Work out the finished part from the listing and answer in its coordinate system (mm). Face numbers are marked on the shaded views. A direction names the side the tool comes from. Round coordinates to 2 decimals unless told otherwise and drop trailing zeros. Order: outer loops, then holes, each group sorted by start corner. A loop starts at its lowest first (then second) coordinate and runs counter-clockwise, first axis right, second up. Notation, with made-up numbers: M 58,38 L 70,38 A15 ccw 70,64 Z; hole C 51,15 d8. An arc over 180 degrees is marked long. Answer as a JSON object with one key per item and string values. Group by question number.
from build123d import *

# Parameters (mm, degrees)
BOSS_EXTRUDE1_DEPTH      = 4.15
BOSS_EXTRUDE1_DEPTH_BACK = 4.15
CUT_EXTRUDE1_DEPTH       = 6
CUT_EXTRUDE1_DEPTH_BACK  = 6
SKETCH2_W                = 10
SKETCH2_H                = 15
CUT_EXTRUDE2_DEPTH       = 2
BOSS_EXTRUDE2_DEPTH      = 2
BOSS_EXTRUDE2_DEPTH_BACK = 2
SKETCH5_W                = 4.4
SKETCH5_H                = 9
CUT_EXTRUDE3_DEPTH       = 3
CUT_EXTRUDE4_DEPTH       = 1
BOSS_EXTRUDE3_DEPTH      = 1
CUT_EXTRUDE5_DEPTH       = 3.2
SKETCH9_W                = 0.8
SKETCH9_H                = 0.8
CUT_EXTRUDE6_DEPTH       = 2.9
SKETCH10_W               = 0.8
SKETCH10_H               = 0.8
CUT_EXTRUDE7_DEPTH       = 2.9
SKETCH11_W               = 0.8
SKETCH11_H               = 0.8
CUT_EXTRUDE8_DEPTH       = 2.9
CUT_EXTRUDE9_DEPTH       = 2.9
CUT_EXTRUDE10_DEPTH      = 2.9
CUT_EXTRUDE11_DEPTH      = 2.9
CUT_EXTRUDE12_DEPTH      = 2.9
CUT_EXTRUDE13_DEPTH      = 2.9
CUT_EXTRUDE14_DEPTH      = 2.9
CUT_EXTRUDE15_DEPTH      = 1.1
BOSS_EXTRUDE4_DEPTH      = 3
BOSS_EXTRUDE4_DEPTH_BACK = 3
SKETCH20_R               = 0.65
BOSS_EXTRUDE5_DEPTH      = 10
SKETCH21_R               = 0.65
BOSS_EXTRUDE6_DEPTH      = 10
CUT_EXTRUDE16_DEPTH      = 3
CUT_EXTRUDE16_DEPTH_BACK = 3


with BuildPart() as part:
    # Sketch1 → Boss-Extrude1 (new, two sides: drawn at the far end of the back side and taken through both)
    with BuildSketch(Plane(origin=(0, 0, 0), x_dir=(0, 0, -1), z_dir=(1, 0, 0)).offset(-BOSS_EXTRUDE1_DEPTH_BACK)):
        with BuildLine():
            Line((-13, 1.4), (-13, -2.4))
            Line((-13, -2.4), (-12.8, -2.6))
            Line((-12.8, -2.6), (-9.85, -2.6))
            Line((-9.85, -2.6), (-9.1, -3.35))
            Line((-9.1, -3.35), (-4, -3.35))
            Line((-4, -3.35), (-4, -2.07))
            Line((-4, -2.07), (-2, -2.07))
            Line((-2, -2.07), (-2, -2.67))
            Line((-2, -2.67), (-0.5, -2.643817403))
            Line((-0.5, -2.643817403), (0, -2.509842806))
            Line((0, -2.509842806), (0, 2.069842806))
            Line((0, 2.069842806), (-0.5, 2.203817403))
            Line((-0.5, 2.203817403), (-2, 2.23))
            Line((-2, 2.23), (-2, 1.6))
            Line((-2, 1.6), (-4, 1.6))
            Line((-4, 1.6), (-4, 2.9))
            ThreePointArc((-4, 2.9), (-6.566392361, 2.777001893), (-9.1, 2.35))
            Line((-9.1, 2.35), (-9.85, 1.6))
            Line((-9.85, 1.6), (-12.8, 1.6))
            Line((-12.8, 1.6), (-13, 1.4))
        make_face()
    extrude(amount=BOSS_EXTRUDE1_DEPTH + BOSS_EXTRUDE1_DEPTH_BACK)

    # Sketch2 → Cut-Extrude1 (cut, two sides: drawn at the far end of the back side and taken through both)
    with BuildSketch(Plane(origin=(0, 0, 0), x_dir=(1, 0, 0), z_dir=(0, 1, 0)).offset(-CUT_EXTRUDE1_DEPTH_BACK)):
        with Locations((0, -6.5)):
            Rectangle(SKETCH2_W, SKETCH2_H)
        Polygon((-4.13, -9.1), (-3.38, -9.85), (-3.38, -12.8), (-3.18, -13), (3.18, -13), (3.38, -12.8), (3.38, -9.85), (4.13, -9.1), (4.13, -4), (3.185, -4), (3.185, -2), (3.8, -2), (3.773817403, -0.5), (3.639842806, 0), (-3.639842806, 0), (-3.773817403, -0.5), (-3.8, -2), (-3.185, -2), (-3.185, -4), (-4.13, -4), align=None, mode=Mode.SUBTRACT)
    extrude(amount=CUT_EXTRUDE1_DEPTH + CUT_EXTRUDE1_DEPTH_BACK, mode=Mode.SUBTRACT)

    # Sketch3 → Cut-Extrude2 (cut)
    with BuildSketch(Plane(origin=(0, 1.6, 0), x_dir=(1, 0, 0), z_dir=(0, 1, 0))):
        Polygon((-2.8, -4), (-2.8, -13), (2.8, -13), (2.8, -4), (2.04, -4), (2.04, 0), (-2.04, 0), (-2.04, -4), align=None)
    extrude(amount=CUT_EXTRUDE2_DEPTH, mode=Mode.SUBTRACT)

    # Sketch4 → Boss-Extrude2 (add, two sides: drawn at the far end of the back side and taken through both)
    with BuildSketch(Plane(origin=(0, 0, 0), x_dir=(0, 0, -1), z_dir=(1, 0, 0)).offset(-BOSS_EXTRUDE2_DEPTH_BACK)):
        with BuildLine():
            Line((-12.51, 3.388062852), (-12.51, 2.87))
            Line((-12.51, 2.87), (-11.612163395, 1.8))
            Line((-11.612163395, 1.8), (-11.312163395, 1.8))
            Line((-11.312163395, 1.8), (-11.411835811, 2.365270364))
            ThreePointArc((-11.411835811, 2.365270364), (-11.368083149, 2.528557522), (-11.214874261, 2.6))
            Line((-11.214874261, 2.6), (-9.35, 2.6))
            ThreePointArc((-9.35, 2.6), (-9.173223305, 2.526776695), (-9.1, 2.35))
            Line((-9.1, 2.35), (-9.1, 1.85))
            ThreePointArc((-9.1, 1.85), (-9.173223305, 1.673223305), (-9.35, 1.6))
            Line((-9.35, 1.6), (-9.35, 0.6))
            Line((-9.35, 0.6), (-7.75, 0.6))
            Line((-7.75, 0.6), (-7.75, 1.6))
            ThreePointArc((-7.75, 1.6), (-7.997487373, 1.702512627), (-8.1, 1.95))
            Line((-8.1, 1.95), (-8.1, 2.25))
            ThreePointArc((-8.1, 2.25), (-7.997487373, 2.497487373), (-7.75, 2.6))
            Line((-7.75, 2.6), (-4, 2.6))
            Line((-4, 2.6), (-4, 4.45))
            Line((-4, 4.45), (-4.8, 4.45))
            ThreePointArc((-4.8, 4.45), (-4.941421356, 4.391421356), (-5, 4.25))
            Line((-5, 4.25), (-5, 4))
            ThreePointArc((-5, 4), (-5.043933983, 3.893933983), (-5.15, 3.85))
            Line((-5.15, 3.85), (-9.1, 3.85))
            ThreePointArc((-9.1, 3.85), (-10.726600682, 3.783744511), (-12.342424242, 3.585417022))
            ThreePointArc((-12.342424242, 3.585417022), (-12.462454663, 3.517513907), (-12.51, 3.388062852))
        make_face()
    extrude(amount=BOSS_EXTRUDE2_DEPTH + BOSS_EXTRUDE2_DEPTH_BACK)

    # Sketch5 → Cut-Extrude3 (cut)
    with BuildSketch(Plane(origin=(0, 1.6, 0), x_dir=(1, 0, 0), z_dir=(0, 1, 0))):
        with Locations((0, -8.3)):
            Rectangle(SKETCH5_W, SKETCH5_H)
        with BuildLine():
            Line((2, -9.1), (2, -4))
            Line((2, -4), (-2, -4))
            Line((-2, -4), (-2, -9.1))
            ThreePointArc((-2, -9.1), (-1.793181663, -10.523168838), (-1.189836183, -11.828602712))
            ThreePointArc((-1.189836183, -11.828602712), (0, -12.5), (1.189836183, -11.828602712))
            ThreePointArc((1.189836183, -11.828602712), (1.793181663, -10.523168838), (2, -9.1))
        make_face(mode=Mode.SUBTRACT)
    extrude(amount=CUT_EXTRUDE3_DEPTH, mode=Mode.SUBTRACT)

    # Sketch6 → Cut-Extrude4 (cut)
    with BuildSketch(Plane(origin=(0, 1.6, 0), x_dir=(1, 0, 0), z_dir=(0, 1, 0))):
        Polygon((-2, -10.5), (-2, -13), (-0.765, -13), (-0.765, -10.7), (0.765, -10.7), (0.765, -13), (2, -13), (2, -10.5), (0.765, -10.5), (0.765, -4), (2, -4), (2, -3), (-2, -3), (-2, -4), (-0.765, -4), (-0.765, -10.5), align=None)
    extrude(amount=CUT_EXTRUDE4_DEPTH, mode=Mode.SUBTRACT)

    # Sketch7 → Boss-Extrude3 (add)
    with BuildSketch(Plane.XY.offset(4)):
        with BuildLine():
            Line((-2.3, -3.35), (-2.190561659, -3.35))
            ThreePointArc((-2.190561659, -3.35), (-2.065337959, -3.394054417), (-1.995280829, -3.50680975))
            ThreePointArc((-1.995280829, -3.50680975), (-1.948171085, -3.597952406), (-1.862068966, -3.653744311))
            ThreePointArc((-1.862068966, -3.653744311), (0, -3.95), (1.862068966, -3.653744311))
            ThreePointArc((1.862068966, -3.653744311), (1.948171087, -3.597952405), (1.99528083, -3.506809747))
            ThreePointArc((1.99528083, -3.506809747), (2.06533796, -3.394054416), (2.190561659, -3.35))
            Line((2.190561659, -3.35), (2.3, -3.35))
            Line((2.3, -3.35), (2, 0))
            Line((2, 0), (-2, 0))
            Line((-2, 0), (-2.3, -3.35))
        make_face()
    extrude(amount=BOSS_EXTRUDE3_DEPTH)

    # Sketch8 → Cut-Extrude5 (cut)
    with BuildSketch(Plane.XY.offset(9.85)):
        Polygon((-1.275, -1.81), (-1.275, -3.41), (1.275, -3.41), (1.275, -1.81), (0.625, -1.81), (0.625, -2.61), (-0.625, -2.61), (-0.625, -1.81), align=None)
    extrude(amount=CUT_EXTRUDE5_DEPTH, mode=Mode.SUBTRACT)

    # Sketch9 → Cut-Extrude6 (cut)
    with BuildSketch(Plane.XY.offset(13)):
        with Locations((-2, -0.01)):
            Rectangle(SKETCH9_W, SKETCH9_H)
    extrude(amount=-CUT_EXTRUDE6_DEPTH, mode=Mode.SUBTRACT)

    # Sketch10 → Cut-Extrude7 (cut)
    with BuildSketch(Plane.XY.offset(13)):
        with Locations((0, -0.01)):
            Rectangle(SKETCH10_W, SKETCH10_H)
    extrude(amount=-CUT_EXTRUDE7_DEPTH, mode=Mode.SUBTRACT)

    # Sketch11 → Cut-Extrude8 (cut)
    with BuildSketch(Plane.XY.offset(13)):
        with Locations((2, -0.01)):
            Rectangle(SKETCH11_W, SKETCH11_H)
    extrude(amount=-CUT_EXTRUDE8_DEPTH, mode=Mode.SUBTRACT)

    # Sketch12 → Cut-Extrude9 (cut)
    with BuildSketch(Plane.XY.offset(13)):
        with BuildLine():
            Line((-2.003613054, -0.76), (-2.996386946, -0.76))
            ThreePointArc((-2.996386946, -0.76), (-2.5, -1.2), (-2.003613054, -0.76))
        make_face()
    extrude(amount=-CUT_EXTRUDE9_DEPTH, mode=Mode.SUBTRACT)

    # Sketch13 → Cut-Extrude10 (cut)
    with BuildSketch(Plane.XY.offset(13)):
        with BuildLine():
            Line((0.003613054, 0.76), (0.996386946, 0.76))
            ThreePointArc((0.996386946, 0.76), (0.5, 1.2), (0.003613054, 0.76))
        make_face()
    extrude(amount=-CUT_EXTRUDE10_DEPTH, mode=Mode.SUBTRACT)

    # Sketch14 → Cut-Extrude11 (cut)
    with BuildSketch(Plane.XY.offset(13)):
        with BuildLine():
            Line((2.003613054, 0.76), (2.996386946, 0.76))
            ThreePointArc((2.996386946, 0.76), (2.5, 1.2), (2.003613054, 0.76))
        make_face()
    extrude(amount=-CUT_EXTRUDE11_DEPTH, mode=Mode.SUBTRACT)

    # Sketch15 → Cut-Extrude12 (cut)
    with BuildSketch(Plane.XY.offset(13)):
        with BuildLine():
            Line((-1.996386946, 0.76), (-1.003613054, 0.76))
            ThreePointArc((-1.003613054, 0.76), (-1.5, 1.2), (-1.996386946, 0.76))
        make_face()
    extrude(amount=-CUT_EXTRUDE12_DEPTH, mode=Mode.SUBTRACT)

    # Sketch16 → Cut-Extrude13 (cut)
    with BuildSketch(Plane.XY.offset(13)):
        with BuildLine():
            Line((-0.003613054, -0.76), (-0.996386946, -0.76))
            ThreePointArc((-0.996386946, -0.76), (-0.5, -1.2), (-0.003613054, -0.76))
        make_face()
    extrude(amount=-CUT_EXTRUDE13_DEPTH, mode=Mode.SUBTRACT)

    # Sketch17 → Cut-Extrude14 (cut)
    with BuildSketch(Plane.XY.offset(13)):
        with BuildLine():
            Line((1.996386946, -0.76), (1.003613054, -0.76))
            ThreePointArc((1.003613054, -0.76), (1.5, -1.2), (1.996386946, -0.76))
        make_face()
    extrude(amount=-CUT_EXTRUDE14_DEPTH, mode=Mode.SUBTRACT)

    # Sketch18 → Cut-Extrude15 (cut)
    with BuildSketch(Plane(origin=(0, -0.56, 0), x_dir=(1, 0, 0), z_dir=(0, 1, 0))):
        Polygon((-2.55, -13), (-2.55, -13.5), (2.55, -13.5), (2.55, -13), (2.05, -12.5), (1.95, -12.5), (1.45, -13), (0.55, -13), (0.05, -12.5), (-0.05, -12.5), (-0.55, -13), (-1.45, -13), (-1.95, -12.5), (-2.05, -12.5), align=None)
    extrude(amount=CUT_EXTRUDE15_DEPTH, mode=Mode.SUBTRACT)

    # Sketch19 → Boss-Extrude4 (add, two sides: drawn at the far end of the back side and taken through both)
    with BuildSketch(Plane(origin=(0, 0, 0), x_dir=(0, 0, -1), z_dir=(1, 0, 0)).offset(-BOSS_EXTRUDE4_DEPTH_BACK)):
        Polygon((-13, 0.54), (-12.85, 0.39), (-8.1, 0.39), (-8.1, -0.41), (-12.85, -0.41), (-13, -0.56), (-8, -0.56), (-8, 0.54), align=None)
    extrude(amount=BOSS_EXTRUDE4_DEPTH + BOSS_EXTRUDE4_DEPTH_BACK)

    # Sketch20 → Boss-Extrude5 (add)
    with BuildSketch(Plane.XY):
        with Locations((2, 0)):
            Circle(SKETCH20_R)
    extrude(amount=-BOSS_EXTRUDE5_DEPTH)

    # Sketch21 → Boss-Extrude6 (add)
    with BuildSketch(Plane.XY):
        with Locations((-2, 0)):
            Circle(SKETCH21_R)
    extrude(amount=-BOSS_EXTRUDE6_DEPTH)

    # Sketch22 → Cut-Extrude16 (cut, two sides: drawn at the far end of the back side and taken through both)
    with BuildSketch(Plane(origin=(0, 0, 0), x_dir=(0, 0, -1), z_dir=(1, 0, 0)).offset(-CUT_EXTRUDE16_DEPTH_BACK)):
        Polygon((8.5, 0.85), (10, -0.65), (10, 0.85), align=None)
    extrude(amount=CUT_EXTRUDE16_DEPTH + CUT_EXTRUDE16_DEPTH_BACK, mode=Mode.SUBTRACT)


solid = part.part
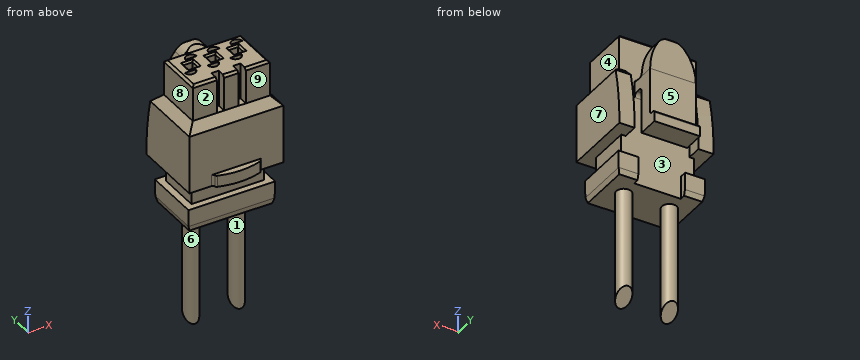
Item 1: A tool of negligible diameter and unlimited length cuts with its end or side. For the marked faces 5, 6, 7, 8 and 9, from which of +Z, -Z, +X, -X, +Y, -Y can it reach the whole face along a straight path? Write none if from no direction.
Item 2: Consider L1, parallel to X at y = -2.25, z = 10 (3 decimals); L2, parallel to Y at x = 0.5, z = 10.25; L3, parallel to Y at x = 1, z = 5.5. Determine where each line is inside the solid, lowest interval first.
Item 3: Each of these flat-tipped pins is pushed along its axis until it touches: pin 1 (1.1 mm diameter, centred on x = 2.5, z = 11, fed in from +Y); pin 2 (4.5 mm diameter, centred on x = 0, z = 8, fed in from +Y); pin 3 (0.9 mm diameter, centred on x = 0, z = 12, fed in from +Y). Where does it stop, or does it pass through?
Item 4: Find section C-C (z = -2.5). Give the vertices of the cut face in (x, y), and give its area (3 significant figures).
Item 5: Find section B-B (y = -3). Give the vertices of the cut face in (x, z).
Item 6: Find section A-A (z = 7.5). Give the vertices of the cut face in (x, y), and give its area (3 significant figures).
Item 7: The mould has two halves that part along X. Classify the marked faces 1, 2, 3 and 4: +X half, -X half, draft (parallel to the pull), parting line (faces both ways), or undercut.
Responses:
{
 "1": {"face 5": "+Z, +X, -X, +Y", "face 6": "-Z", "face 7": "+Z, -Z, +X, +Y, -Y", "face 8": "+Z, -X, +Y, -Y", "face 9": "+Z, +X, -X, -Y"},
 "2": {"L1": "x = -3.38 to -1.275, -0.625 to 0.625, 1.275 to 3.38", "L2": "y = -2.6 to 0.76, 1.2 to 1.6, 2.6 to 3.82", "L3": "y = -3.35 to 1.6, 2.6 to 3.85"},
 "3": {"pin 1": "stops at y = 1.6", "pin 2": "stops at y = 3.85", "pin 3": "stops at y = 3.7"},
 "4": {"outline": "C -2,0 d1.3; C 2,0 d1.3", "area": "2.65 mm^2"},
 "5": {"outline": "M -4.13,4 L 4.13,4 L 4.13,9.1 L 3.78,9.45 L -3.78,9.45 L -4.13,9.1 Z"},
 "6": {"outline": "M -4.13,-3.35 L 4.13,-3.35 L 4.13,2.66 L 2.8,2.66 L 2.8,1.6 L -2.8,1.6 L -2.8,2.66 L -4.13,2.66 Z; M -2,2.6 L 2,2.6 L 2,3.85 L -2,3.85 Z", "area": "48.7 mm^2"},
 "7": {"face 1": "undercut", "face 2": "draft", "face 3": "undercut", "face 4": "+X half"}
}
